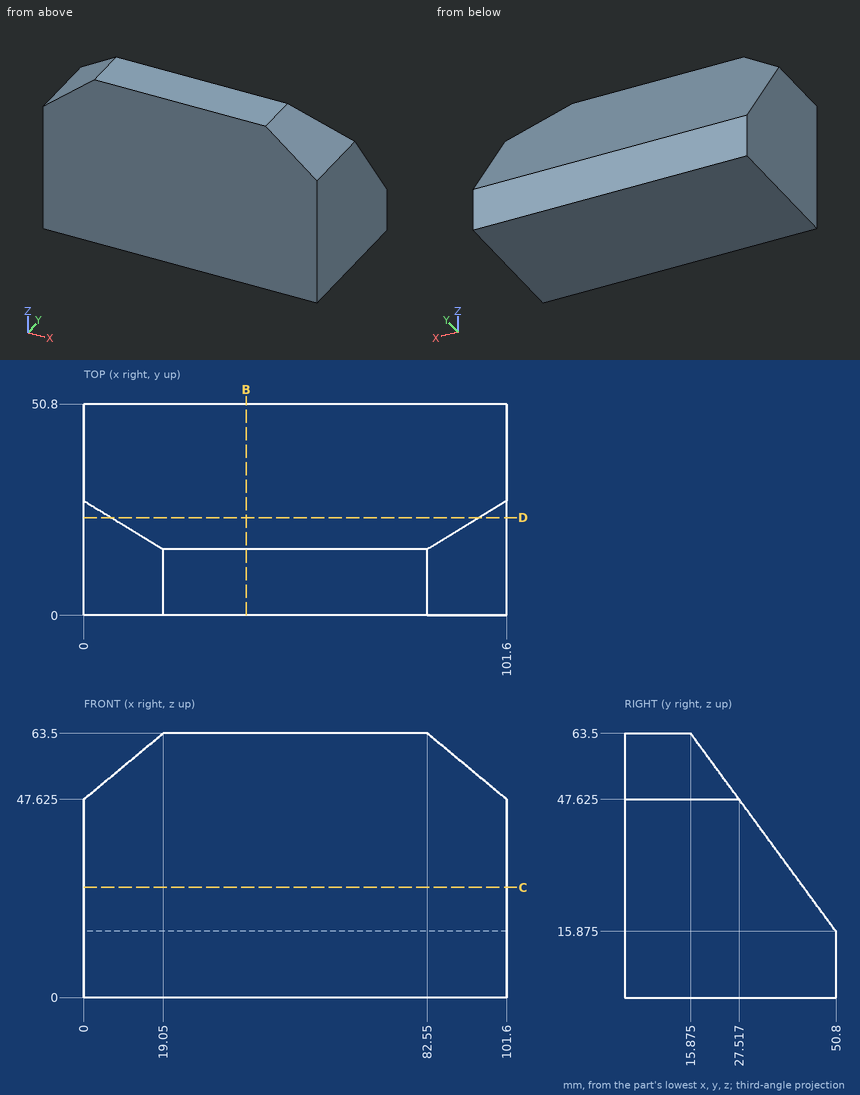
For this review, use the dimensioned drawing (mm, ordinates from the lowest corner) and the shaded views. Round coordinates to 2 decimals unless told otherwise and drop trailing zeros. Write each loop counter-clockwise with the first axis right and the second up, starting at its lowest first coordinate (ties: lowest second). Pieces come first, ordered by that corner, then holes. Notation, with made-up numbers: (5, -27.5) -> (14, -27.5) arc R12 ccw to (14, -12.5) -> close; hole circle Ø2 at (25, -10). An arc over 180 degrees is marked (long way). Use one line per item in the form item = value.
Q1. Consider section B-B (x = 39). State the section outline as (y, z) points (1 decimal).
Resolved:
outline = (0, 0) -> (50.8, 0) -> (50.8, 15.9) -> (15.9, 63.5) -> (0, 63.5) -> close
Q2. Consider section D-D (y = 23.5). State the section outline as (x, z) points (1 decimal), then the cut area to 3 significant figures.
Resolved:
outline = (0, 0) -> (101.6, 0) -> (101.6, 47.6) -> (95, 53.1) -> (6.6, 53.1) -> (0, 47.6) -> close
area = 5,360 mm²
Q3. To check wall thickness, follow probe 1 along Z at (x, y) = (30, 27); probe 2 along Y at (x, z) = (89.5, 27.5) (1 decimal); probe 3 along Z at (x, y) = (32, 16). State the ranges of each line that lie inside material, in increasing order. Write a range as from..to.
Resolved:
probe_1 = 0..48.33
probe_2 = 0..42.3
probe_3 = 0..63.33
Q4. Consider section C-C (z = 26.5). State the section outline as (x, y) points.
Resolved:
outline = (0, 0) -> (101.6, 0) -> (101.6, 43.01) -> (0, 43.01) -> close
Q5. Clearance check with flat-ended pins moving along their axes: pin 1 Ø3 at (y, z) = (40, 35.5) entering from +X; pin 2 Ø2 at (x, y) = (80.5, 19.5) entering from +Z. State where each tip first meets the part, or that it passes through.
Resolved:
pin_1 = through
pin_2 = 59.92
